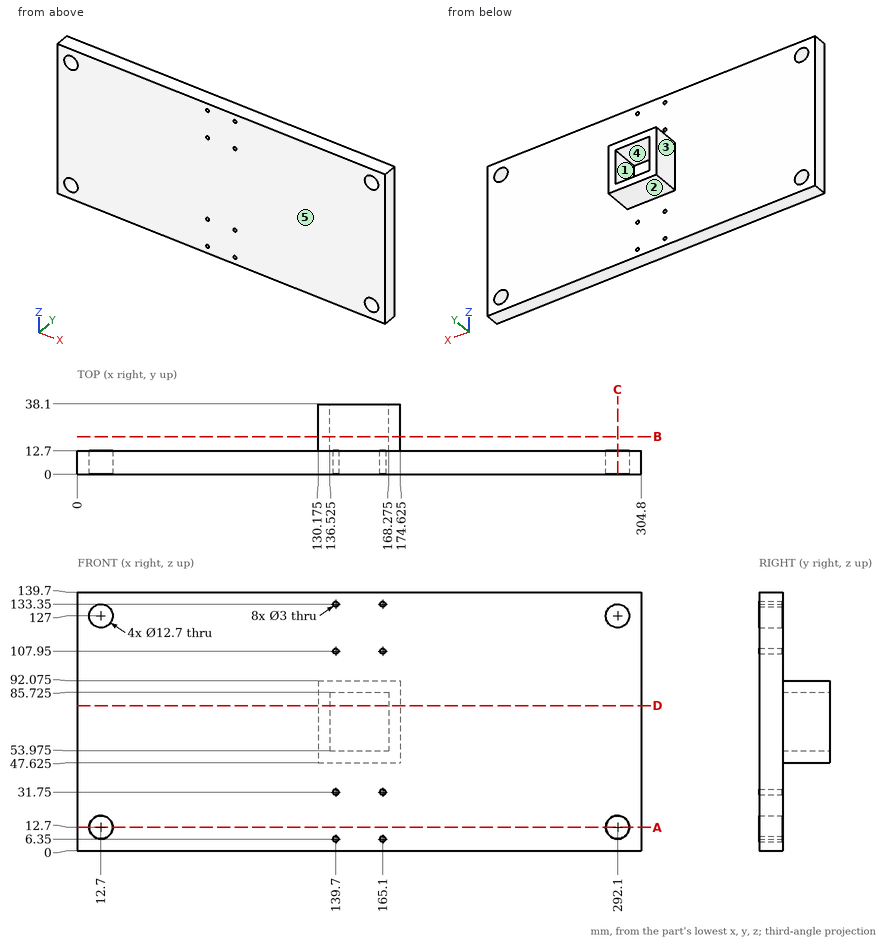
Job drawing, mm, ordinate dimensions from the low corner. One solid piece. A direction names the side the tool comes from. Coordinates: 2 decimals unless noted, no trailing zeros. Write each loop counter-clockwise with the first axis right and the second up, starting at its lowest first coordinate (ties: lowest second). Pieces come first, ordered by that corner, then holes.
Item 1: Slice it at D-D (z = 78.5). Write the cut outline in (x, y) (3 decimals), and give its area (3 significant figures).
Item 2: Mould opens along X. For the marked faces 1, 2 and 3 say: released by +X, released by -X, zero draft, split by the parting line, or undercut.
Item 3: Slice it at B-B (y = 20.5). Write the cut outline in (x, z) (3 decimals).
Item 4: Pin check, flat tips, straight feed: pin 1 (4 mm diameter, centred on x = 165.1, z = 6.35, fed in from +Y); pin 2 (7.5 mm diameter, centred on x = 159.5, y = 30.5, fed in from +Z) (3 decimals); pin 3 (1 mm diameter, centred on y = 20, z = 87.5, fed in from +X) (3 decimals). Stop position of each tip, or through.
Item 5: Probe line 1 (Z direction, x = 292.1, y = 6.5); line 2 (Z direction, x = 139.7, y = 3.25); line 3 (X direction, y = 5, z = 107). List the from-to ranges inside material, lowest first.
Item 6: Slice it at A-A (z = 12.7). Write the cut outline in (x, y), and give its area (3 significant figures).
Item 7: Which spindle directions (+Z, -Z, +X, -X, +Y, -Y) get a long thin tool onto all of the face, cutting with end or side? Do the marked faces 4 and 5. Say none if no direction does.
Item 8: Slice it at C-C (x = 292.1). Write the cut outline in (y, z).
Results found:
1. outline: (0, 0) - (304.8, 0) - (304.8, 12.7) - (174.625, 12.7) - (174.625, 38.1) - (168.275, 38.1) - (168.275, 12.7) - (136.525, 12.7) - (136.525, 38.1) - (130.175, 38.1) - (130.175, 12.7) - (0, 12.7) - close
1. area: 4,190 mm2
2. face 1: undercut
2. face 2: zero draft
2. face 3: released by -X
3. outline: (130.175, 47.625) - (174.625, 47.625) - (174.625, 92.075) - (130.175, 92.075) - close; hole (136.525, 53.975) - (168.275, 53.975) - (168.275, 85.725) - (136.525, 85.725) - close
4. pin 1: stops at y = 12.7
4. pin 2: stops at z = 92.075
4. pin 3: stops at x = 174.625
5. line 1: z = 0 to 6.35, 19.05 to 120.65, 133.35 to 139.7
5. line 2: z = 0 to 4.85, 7.85 to 30.25, 33.25 to 106.45, 109.45 to 131.85, 134.85 to 139.7
5. line 3: x = 0 to 138.54, 140.86 to 163.94, 166.26 to 304.8
6. outline: (0, 0) - (6.35, 0) - (6.35, 12.7) - (0, 12.7) - close; (19.05, 0) - (285.75, 0) - (285.75, 12.7) - (19.05, 12.7) - close; (298.45, 0) - (304.8, 0) - (304.8, 12.7) - (298.45, 12.7) - close
6. area: 3,550 mm2
7. face 4: +Y
7. face 5: +Z, -Z, +X, -X, -Y
8. outline: (0, 0) - (12.7, 0) - (12.7, 6.35) - (0, 6.35) - close; (0, 19.05) - (12.7, 19.05) - (12.7, 120.65) - (0, 120.65) - close; (0, 133.35) - (12.7, 133.35) - (12.7, 139.7) - (0, 139.7) - close
